Work out the finished part from the listing and answer in its coordinate system (mm). Face numbers are marked on the shaded views. A direction names the side the tool comes from. Give positions to 0.01 mm unless a question says otherwise; leave off trailing zeros. Loops run counter-clockwise (first coordinate to the right, second up) from the corner with the lowest first, then second, coordinate; pieces in that order, holes last. Notation, with made-up numbers: (61.25, 13) - (104.25, 13) arc R25 cw to (104.25, 51) - close; hole circle Ø9 at (53.25, -16). An arc over 180 degrees is marked (long way). Use CSV: the item, a comma, the result in double quotes.
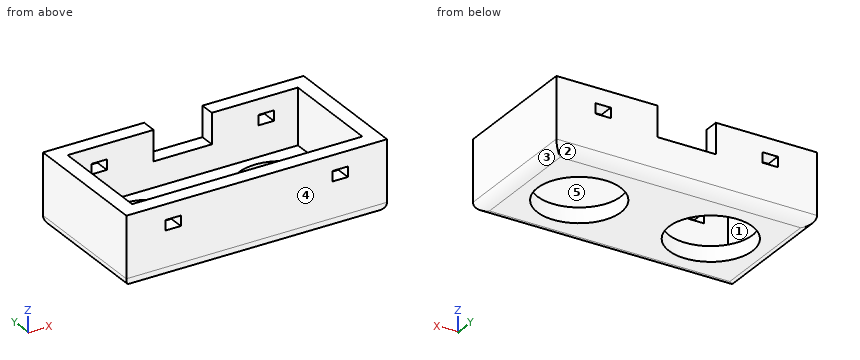
Autodesk Fusion 360 part; units mm, degrees
sketch "Sketch1" plane through (0, 0, 0) normal (0, 0, 1) x (1, 0, 0)
  line L0 (0, 0) -> (51.5, 0)
  line L1 (51.5, 0) -> (51.5, 26.5)
  line L2 (51.5, 26.5) -> (0, 26.5)
  line L3 (0, 26.5) -> (0, 0)
  line L4 (3, 3) -> (48.5, 3)
  line L5 (48.5, 3) -> (48.5, 23.5)
  line L6 (48.5, 23.5) -> (3, 23.5)
  line L7 (3, 23.5) -> (3, 3)
  circle A0 centre (12.75, 13.25) radius 8.25
  circle A1 centre (38.75, 13.25) radius 8.25
  dimension "d1" = 51.5
  dimension "d2" = 26.5
  dimension "d3" = -3
  dimension "d4" = 16.5
  dimension "d5" = 16.5
  dimension "d6" = 26
  dimension "d7" = 13.25
  dimension "d8" = 12.75
extrude "Extrude1" add sketch "Sketch1" along normal blind 3 contours L4 L5 L6 L7
extrude "Extrude2" add sketch "Sketch1" along normal blind 14 contours L0 L1 L2 L3
sketch "Sketch2" plane through (0, 0, 14) normal (0, 0, 1) x (-1, 0, 0)
  line L0 (-3, -3) -> (-3, -23.5)
  line L1 (-3, -23.5) -> (-48.5, -23.5)
  line L2 (-48.5, -23.5) -> (-48.5, -3)
  line L3 (-48.5, -3) -> (-3, -3)
  line L4 (0, -26.5) -> (0, 0)
  line L5 (0, 0) -> (-51.5, 0)
  line L6 (-51.5, 0) -> (-51.5, -26.5)
  line L7 (-51.5, -26.5) -> (0, -26.5)
  line L8 (-20, -26.5) -> (-31.5, -26.5)
  line L9 (-31.5, -26.5) -> (-31.5, -23.5)
  line L10 (-31.5, -23.5) -> (-20, -23.5)
  line L11 (-20, -23.5) -> (-20, -26.5)
  dimension "d13" = 20
  dimension "d14" = 20
extrude "Extrude3" cut sketch "Sketch2" against normal blind 6 contours L1 L7 L8 L9 L10 L11
sketch "Sketch3" plane through (0, 0, 0) normal (0, -1, 0) x (1, 0, 0)
  line L0 (0, 0) -> (51.5, 0)
  line L1 (51.5, 0) -> (51.5, 14)
  line L2 (51.5, 14) -> (0, 14)
  line L3 (0, 14) -> (0, 0)
  line L4 (7.75, 11) -> (10.75, 11)
  line L5 (10.75, 11) -> (10.75, 9)
  line L6 (10.75, 9) -> (7.75, 9)
  line L7 (7.75, 9) -> (7.75, 11)
  line L8 (40.75, 11) -> (43.75, 11)
  line L9 (43.75, 11) -> (43.75, 9)
  line L10 (43.75, 9) -> (40.75, 9)
  line L11 (40.75, 9) -> (40.75, 11)
  dimension "d18" = 3
  dimension "d19" = 2
  dimension "d20" = 30
  dimension "d21" = 51.5
  dimension "d22" = 10.75
  dimension "d23" = 3
extrude "Extrude4" cut sketch "Sketch3" against normal up to surface (26.5 mm away) contours L4 L5 L6 L7 | L8 L9 L10 L11
fillet "Fillet1" radius 2 4 edges at (25.75, 0, 0) (0, 13.25, 0) (25.75, 26.5, 0) (51.5, 13.25, 0)
equation "d1 = 45 mm + 3 mm + 3 mm + 0.5 mm"
equation "d2 = 20 mm + 3 mm + 3 mm + 0.5 mm"
equation "d4 = 16 mm + 0.5 mm"
equation "d5 = 16 mm + 0.5 mm"
equation "d7 = d2 / 2"
equation "d8 = ( d1 - d6 ) / 2"
equation "d11 = 10 mm + 3 mm + 1 mm"
equation "d14 = d13"
equation "d22 = ( d21 - d20 ) / 2"
Item 1: The mould has two halves that part along Y. Classify the marked faces 3, 4 and 5: pulls with the +Y half, pulls with the -Y half, needs draft (parallel to the pull), parting line crosses it, or undercut.
Determined:
face 3,"needs draft"
face 4,"pulls with the -Y half"
face 5,"undercut"
Item 2: A cutting plane is placed at B-B on z = 3.75. Determine the outline of the cut face in (x, y).
Determined:
outline,"(0, 0) - (51.5, 0) - (51.5, 26.5) - (0, 26.5) - close; hole (3, 3) - (48.5, 3) - (48.5, 23.5) - (3, 23.5) - close"
Item 3: A cutting plane is placed at D-D on y = 2.5. Determine the outline of the cut face in (x, z).
Determined:
outline,"(0, 2) arc R2 ccw to (2, 0) - (49.5, 0) arc R2 ccw to (51.5, 2) - (51.5, 14) - (0, 14) - close; hole (7.75, 9) - (10.75, 9) - (10.75, 11) - (7.75, 11) - close; hole (40.75, 9) - (43.75, 9) - (43.75, 11) - (40.75, 11) - close"
Item 4: A cutting plane is placed at C-C on x = 38.75. Determine the outline of the cut face in (y, z).
Determined:
outline,"(0, 2) arc R2 ccw to (2, 0) - (5, 0) - (5, 3) - (3, 3) - (3, 14) - (0, 14) - close; (21.5, 0) - (24.5, 0) arc R2 ccw to (26.5, 2) - (26.5, 14) - (23.5, 14) - (23.5, 3) - (21.5, 3) - close"
Item 5: For the marked faces 1 and 2, determine the directions among +Z, -Z, +X, -X, +Y, -Y from which every point of the face is accessible in a straight line to the end or side of a thin tool.
Determined:
face 1,"+Z"
face 2,"-Z, +X, -X, +Y"
Item 6: Find the intervals of material crossed by line 1 (X direction, y = 8, z = 10.25); line 2 (Y direction, x = 12, z = 12.75); line 3 (Y direction, x = 26.5, z = 9), in increasing order.
Determined:
line 1,"x = 0 to 3, 48.5 to 51.5"
line 2,"y = 0 to 3, 23.5 to 26.5"
line 3,"y = 0 to 3"
Item 7: Given P1, Ø5, axis at y = 3.5, z = 2, coming from the -X side; P2, Ø0.9, axis at x = 10, y = 25.5, coming from the -Z side; P3, Ø8, axis at x = 36.5, y = 17, coming from the +Z side, each flat-ended and moving along its own axis, determine where each tip first touches the part or whether it passes through.
Determined:
P1,"stops at x = 0"
P2,"stops at z = 0.08"
P3,"stops at z = 3"
Item 8: A cutting plane is placed at A-A on y = 13.25. Determine the outline of the cut face in (x, z).
Determined:
outline,"(0, 2) arc R2 ccw to (2, 0) - (4.5, 0) - (4.5, 3) - (3, 3) - (3, 14) - (0, 14) - close; (21, 0) - (30.5, 0) - (30.5, 3) - (21, 3) - close; (47, 0) - (49.5, 0) arc R2 ccw to (51.5, 2) - (51.5, 14) - (48.5, 14) - (48.5, 3) - (47, 3) - close"
